Could you check a few things on this model? Use its own coordinates, in mm. A direction names the side the tool comes from. Coordinates: 2 decimals unless noted, no trailing zeros. Loops run counter-clockwise (first coordinate to the right, second up) from the corner with the lowest first, then second, coordinate; pieces in that order, holes last.
1) Imagine slicing it at B-B on z = 13.5. Give the number of separate pieces and of enclosed holes in the cut face, plus the area to 3 significant figures.
2) For faces 1 (the face through (-90, -99.698, 2)), 2 (the face through (21.213, -128, 2)), 3 (the face through (-69, -60.5, 25)), 4 (the face through (-40, -159.697, 2)), which set-ups out of +Z, -Z, +X, -X, +Y, -Y let a thin tool reach every point of the face, with its end or its side?
3) If I drill on line 1 along Y through (x, z) = (-30, 30); line 2 along X through (y, z) = (-40.5, 17.5); line 3 along Y through (x, z) = (1.5, 4.5), over which ranges is the centre line in solid material (lowest first)?
4) Thinking about a two-plate mould opening in X: for faces 5 (the face through (19, -45, 45.5)), 6 (the face through (-10, -3, 25)), 7 (the face through (-40, -3, 25)), 8 (the face through (6.972, -176.369, 2.465)), which applies, released by +X, released by -X, zero draft, split by the parting line, or undercut?
5) Imagine slicing it at A-A on y = -82.5. Please give me the cut outline in (x, z), plus the area to 3 significant figures.
6) Will these pins go through, and if not, where does the flat tip stop? P1, Ø1.2, axis at x = -98.5, z = 1.5, coming from the -Y side; P2, Ø5.5, axis at x = -52, z = 1.5, coming from the -Y side; P3, Ø4, axis at y = -119.5, z = 3.5, coming from the -X side; P4, Ø1.8, axis at x = -96.7, y = -77.2, coming from the -Z side.
```python
from build123d import *

# Parameters (mm, degrees)
DODANIE_WYCI_GNI_CIE1_DEPTH     = 5
WYTNIJ_WYCI_GNI_CIE3_DEPTH      = 16
WYTNIJ_WYCI_GNI_CIE3_DEPTH_BACK = 4
SZKIC3_R                        = 0.8
WYTNIJ_WYCI_GNI_CIE4_DEPTH      = 26
WYTNIJ_WYCI_GNI_CIE4_DEPTH_BACK = 52
SZKIC5_R                        = 1.5
WYTNIJ_WYCI_GNI_CIE5_DEPTH      = 31
WYTNIJ_WYCI_GNI_CIE5_DEPTH_BACK = 69
WYTNIJ_WYCI_GNI_CIE6_DEPTH      = 22
WYTNIJ_WYCI_GNI_CIE6_DEPTH_BACK = 83
SZKIC7_R                        = 1
SZKIC8_W                        = 30
SZKIC8_H                        = 5
DODANIE_WYCI_GNI_CIE2_DEPTH     = 45.5
SZKIC10_W                       = 30
SZKIC10_H                       = 5
DODANIE_WYCI_GNI_CIE3_DEPTH     = 40.5
WYTNIJ_WYCI_GNI_CIE7_DEPTH      = 112
WYTNIJ_WYCI_GNI_CIE7_DEPTH_BACK = 158
SZKIC11_R                       = 0.75
WYTNIJ_WYCI_GNI_CIE8_DEPTH      = 220
WYTNIJ_WYCI_GNI_CIE8_DEPTH_BACK = 402
SZKIC12_R                       = 0.75
SZKIC13_W                       = 5
SZKIC13_H                       = 30
DODANIE_WYCI_GNI_CIE4_DEPTH     = 40.5
WYTNIJ_WYCI_GNI_CIE9_DEPTH      = 48
WYTNIJ_WYCI_GNI_CIE9_DEPTH_BACK = 85
SZKIC14_R                       = 0.75


with BuildPart() as part:
    # Szkic1 → Dodanie-wyciągnięcie1 (new body)
    with BuildSketch(Plane.XY):
        Polygon((0, 0), (-50, 0), (-64.142135624, 14.142135624), (-71.213203436, 7.071067812), (-68.384776311, 4.242640687), (-75.455844123, -2.828427125), (-78.284271247, 0), (-85.355339059, -7.071067812), (-71.213203436, -21.213203436), (-71.213203436, -61.213203436), (-79.69848481, -69.69848481), (-99.69848481, -69.69848481), (-99.69848481, -79.69848481), (-95.69848481, -79.69848481), (-95.69848481, -89.69848481), (-99.69848481, -89.69848481), (-99.69848481, -99.69848481), (-79.69848481, -99.69848481), (-71.213203436, -108.183766184), (-71.213203436, -148.183766184), (-85.355339059, -162.325901808), (-78.284271247, -169.39696962), (-75.455844123, -166.568542495), (-68.384776311, -173.639610307), (-71.213203436, -176.468037432), (-64.142135624, -183.539105243), (-50, -169.39696962), (0, -169.39696962), (14.142135624, -183.539105243), (21.213203436, -176.468037432), (18.384776311, -173.639610307), (25.455844123, -166.568542495), (28.284271247, -169.39696962), (35.355339059, -162.325901808), (21.213203436, -148.183766184), (21.213203436, -108.183766184), (29.69848481, -99.69848481), (49.69848481, -99.69848481), (49.69848481, -89.69848481), (45.69848481, -89.69848481), (45.69848481, -79.69848481), (49.69848481, -79.69848481), (49.69848481, -69.69848481), (29.69848481, -69.69848481), (21.213203436, -61.213203436), (21.213203436, -21.213203436), (35.355339059, -7.071067812), (28.284271247, 0), (25.455844123, -2.828427125), (18.384776311, 4.242640687), (21.213203436, 7.071067812), (14.142135624, 14.142135624), align=None)
    extrude(amount=DODANIE_WYCI_GNI_CIE1_DEPTH)

    # Szkic3 → Wytnij-wyciągnięcie3 (cut, two sides: drawn at the far end of the back side and taken through both)
    with BuildSketch(Plane.XY.offset(-WYTNIJ_WYCI_GNI_CIE3_DEPTH_BACK)):
        with Locations((31.69848481, -77.19848481)):
            Circle(SZKIC3_R)
        with Locations((46.69848481, -77.19848481)):
            Circle(SZKIC3_R)
        with Locations((31.69848481, -92.19848481)):
            Circle(SZKIC3_R)
        with Locations((46.69848481, -92.19848481)):
            Circle(SZKIC3_R)
        with Locations((-81.69848481, -77.19848481)):
            Circle(SZKIC3_R)
        with Locations((-96.69848481, -77.19848481)):
            Circle(SZKIC3_R)
        with Locations((17.324116139, -154.901280605)):
            Circle(SZKIC3_R)
        with Locations((27.930717857, -165.507882323)):
            Circle(SZKIC3_R)
        with Locations((17.324116139, -176.114484041)):
            Circle(SZKIC3_R)
        with Locations((6.717514421, -165.507882323)):
            Circle(SZKIC3_R)
        with Locations((-67.324116139, -154.901280605)):
            Circle(SZKIC3_R)
        with Locations((-77.930717857, -165.507882323)):
            Circle(SZKIC3_R)
        with Locations((-67.324116139, -176.114484041)):
            Circle(SZKIC3_R)
        with Locations((-56.717514421, -165.507882323)):
            Circle(SZKIC3_R)
        with Locations((17.324116139, 6.717514421)):
            Circle(SZKIC3_R)
        with Locations((27.930717857, -3.889087297)):
            Circle(SZKIC3_R)
        with Locations((6.717514421, -3.889087297)):
            Circle(SZKIC3_R)
        with Locations((17.324116139, -14.495689014)):
            Circle(SZKIC3_R)
        with Locations((-67.324116139, 6.717514421)):
            Circle(SZKIC3_R)
        with Locations((-56.717514421, -3.889087297)):
            Circle(SZKIC3_R)
        with Locations((-77.930717857, -3.889087297)):
            Circle(SZKIC3_R)
        with Locations((-67.324116139, -14.495689014)):
            Circle(SZKIC3_R)
        with Locations((-96.69848481, -92.19848481)):
            Circle(SZKIC3_R)
        with Locations((-81.69848481, -92.19848481)):
            Circle(SZKIC3_R)
    extrude(amount=WYTNIJ_WYCI_GNI_CIE3_DEPTH + WYTNIJ_WYCI_GNI_CIE3_DEPTH_BACK, mode=Mode.SUBTRACT)

    # Szkic5 → Wytnij-wyciągnięcie4 (cut, two sides: drawn at the far end of the back side and taken through both)
    with BuildSketch(Plane.XY.offset(-WYTNIJ_WYCI_GNI_CIE4_DEPTH_BACK)):
        with Locations((-60.003203436, -26.5)):
            Circle(SZKIC5_R)
        with Locations((9.996796564, -26.5)):
            Circle(SZKIC5_R)
        with Locations((9.996796564, -106.5)):
            Circle(SZKIC5_R)
        with Locations((-60.003203436, -106.5)):
            Circle(SZKIC5_R)
        Polygon((4.496796564, -21.5), (-54.503203436, -21.5), (-54.503203436, -32), (-65.003203436, -32), (-65.003203436, -101), (-54.503203436, -101), (-54.503203436, -111.5), (4.496796564, -111.5), (4.496796564, -101), (14.996796564, -101), (14.996796564, -32), (4.496796564, -32), align=None)
    extrude(amount=WYTNIJ_WYCI_GNI_CIE4_DEPTH + WYTNIJ_WYCI_GNI_CIE4_DEPTH_BACK, mode=Mode.SUBTRACT)

    # Szkic6 → Wytnij-wyciągnięcie5 (cut, two sides: drawn at the far end of the back side and taken through both)
    with BuildSketch(Plane.XY.offset(5).offset(-WYTNIJ_WYCI_GNI_CIE5_DEPTH_BACK)):
        Polygon((-30.913203436, -116.49696962), (-49.713203436, -116.49696962), (-49.713203436, -121.49696962), (-57.713203436, -121.49696962), (-57.713203436, -154.69696962), (-49.713203436, -154.69696962), (-49.713203436, -159.69696962), (-30.913203436, -159.69696962), (-30.913203436, -154.69696962), (-25.913203436, -154.69696962), (-25.913203436, -121.49696962), (-30.913203436, -121.49696962), align=None)
        Polygon((-0.286796564, -121.49696962), (-0.286796564, -116.49696962), (-19.086796564, -116.49696962), (-19.086796564, -121.49696962), (-24.086796564, -121.49696962), (-24.086796564, -154.69696962), (-19.086796564, -154.69696962), (-19.086796564, -159.69696962), (-0.286796564, -159.69696962), (-0.286796564, -154.69696962), (7.713203436, -154.69696962), (7.713203436, -121.49696962), align=None)
    extrude(amount=WYTNIJ_WYCI_GNI_CIE5_DEPTH + WYTNIJ_WYCI_GNI_CIE5_DEPTH_BACK, mode=Mode.SUBTRACT)

    # Szkic7 → Wytnij-wyciągnięcie6 (cut, two sides: drawn at the far end of the back side and taken through both)
    with BuildSketch(Plane.XY.offset(5).offset(-WYTNIJ_WYCI_GNI_CIE6_DEPTH_BACK)):
        with Locations((-53.513203436, -118.69696962)):
            Circle(SZKIC7_R)
        with Locations((-28.113203436, -118.69696962)):
            Circle(SZKIC7_R)
        with Locations((-21.886796564, -118.69696962)):
            Circle(SZKIC7_R)
        with Locations((3.513203436, -118.69696962)):
            Circle(SZKIC7_R)
        with Locations((3.513203436, -157.49696962)):
            Circle(SZKIC7_R)
        with Locations((-21.886796564, -157.49696962)):
            Circle(SZKIC7_R)
        with Locations((-28.113203436, -157.49696962)):
            Circle(SZKIC7_R)
        with Locations((-53.513203436, -157.49696962)):
            Circle(SZKIC7_R)
    extrude(amount=WYTNIJ_WYCI_GNI_CIE6_DEPTH + WYTNIJ_WYCI_GNI_CIE6_DEPTH_BACK, mode=Mode.SUBTRACT)

    # Szkic8 → Dodanie-wyciągnięcie2 (add)
    with BuildSketch(Plane.XY):
        with Locations((-25, -2.5)):
            Rectangle(SZKIC8_W, SZKIC8_H)
    extrude(amount=DODANIE_WYCI_GNI_CIE2_DEPTH)

    # Szkic10 → Dodanie-wyciągnięcie3 (add)
    with BuildSketch(Plane.XY.offset(5)):
        with Locations((-25, -166.89696962)):
            Rectangle(SZKIC10_W, SZKIC10_H)
    extrude(amount=DODANIE_WYCI_GNI_CIE3_DEPTH)

    # Szkic11 → Wytnij-wyciągnięcie7 (cut, two sides: drawn at the far end of the back side and taken through both)
    with BuildSketch(Plane.XY.offset(45.5).offset(-WYTNIJ_WYCI_GNI_CIE7_DEPTH_BACK)):
        with Locations((-30, -2.5)):
            Circle(SZKIC11_R)
        with Locations((-20, -2.5)):
            Circle(SZKIC11_R)
    extrude(amount=WYTNIJ_WYCI_GNI_CIE7_DEPTH + WYTNIJ_WYCI_GNI_CIE7_DEPTH_BACK, mode=Mode.SUBTRACT)

    # Szkic12 → Wytnij-wyciągnięcie8 (cut, two sides: drawn at the far end of the back side and taken through both)
    with BuildSketch(Plane.XY.offset(45.5).offset(-WYTNIJ_WYCI_GNI_CIE8_DEPTH_BACK)):
        with Locations(Location((-30, -166.89696962, 0), (0, 0, 180))):
            Circle(SZKIC12_R)
        with Locations(Location((-20, -166.89696962, 0), (0, 0, 180))):
            Circle(SZKIC12_R)
    extrude(amount=WYTNIJ_WYCI_GNI_CIE8_DEPTH + WYTNIJ_WYCI_GNI_CIE8_DEPTH_BACK, mode=Mode.SUBTRACT)

    # Szkic13 → Dodanie-wyciągnięcie4 (add)
    with BuildSketch(Plane.XY.offset(5)):
        with Locations((-68.713203436, -45.5)):
            Rectangle(SZKIC13_W, SZKIC13_H)
        with Locations((18.713203436, -45.5)):
            Rectangle(SZKIC13_W, SZKIC13_H)
    extrude(amount=DODANIE_WYCI_GNI_CIE4_DEPTH)

    # Szkic14 → Wytnij-wyciągnięcie9 (cut, two sides: drawn at the far end of the back side and taken through both)
    with BuildSketch(Plane.XY.offset(-WYTNIJ_WYCI_GNI_CIE9_DEPTH_BACK)):
        with Locations(Location((-68.713203436, -40.5, 0), (0, 0, 180))):
            Circle(SZKIC14_R)
        with Locations(Location((-68.713203436, -50.5, 0), (0, 0, 180))):
            Circle(SZKIC14_R)
        with Locations((18.713203436, -40.5)):
            Circle(SZKIC14_R)
        with Locations((18.713203436, -50.5)):
            Circle(SZKIC14_R)
    extrude(amount=WYTNIJ_WYCI_GNI_CIE9_DEPTH + WYTNIJ_WYCI_GNI_CIE9_DEPTH_BACK, mode=Mode.SUBTRACT)


solid = part.part
```
Filled in:
1. separate pieces: 4
1. enclosed holes: 8
1. area: 586 mm2
2. face 1: +Z, -Z, -X
2. face 2: +Z, -Z, +X
2. face 3: +Z, +X, -X, -Y
2. face 4: +Z, -Z
3. line 1: y = -169.4 to -167.65, -166.15 to -164.4, -5 to -3.25, -1.75 to 0
3. line 2: x = -71.21 to -69.46, -67.96 to -66.21, 16.21 to 17.96, 19.46 to 21.21
3. line 3: y = -170.9 to -154.7, -121.5 to -111.5, -21.5 to 1.5
4. face 5: zero draft
4. face 6: released by +X
4. face 7: released by -X
4. face 8: undercut
5. outline: (-95.7, 0) - (-65, 0) - (-65, 5) - (-95.7, 5) - close; (15, 0) - (45.7, 0) - (45.7, 5) - (15, 5) - close
5. area: 307 mm2
6. P1: stops at y = -99.7
6. P2: stops at y = -174.15
6. P3: stops at x = -71.21
6. P4: stops at z = 0
